```python
from build123d import *

# Parameters (mm, degrees)
MAIN_DEPTH            = 5
GEAR_AXIS_HOLES_D     = 5.5
FILLET1_R             = 3
F_3_CLEARANCE_HOLE1_D = 2.794


with BuildPart() as part:
    # Base → Main (new body)
    with BuildSketch(Plane.XY):
        Polygon((0, 27.5), (-33, 27.5), (-33, -27.5), (0, -27.5), (0, -40.995), (24, -40.995), (31.5, -40.995), (31.5, 27.5), (24, 27.5), align=None)
    extrude(amount=MAIN_DEPTH)

    # Gear Axis Holes (through all)
    with Locations(Plane(origin=(0, 0, 0), x_dir=(-1, 0, 0), z_dir=(0, 0, -1))):
        with Locations((23, -20), (23, 20)):
            Hole(GEAR_AXIS_HOLES_D / 2)

    # Fillet1
    fillet1_edges = [part.edges().sort_by_distance(p)[0] for p in [
        (31.5, 27.5, 2.5),
        (31.5, -40.995, 2.5),
        (0, -40.995, 2.5),
        (0, -27.5, 2.5),
        (-33, -27.5, 2.5),
        (-33, 27.5, 2.5),
    ]]
    fillet(fillet1_edges, radius=FILLET1_R)

    # #3 Clearance Hole1 (through all)
    with Locations(Plane.XY.offset(5)):
        with Locations((10, 23.75), (27.75, 23.75), (27.75, -37.245), (10, -37.245)):
            Hole(F_3_CLEARANCE_HOLE1_D / 2)


solid = part.part
```
Can you work these out from the model? Positions are in its coordinate system, mm. A direction names the side the tool comes from. Round coordinates to 2 decimals unless told otherwise and drop trailing zeros. Loops run counter-clockwise (first coordinate to the right, second up) from the corner with the lowest first, then second, coordinate; pieces in that order, holes last. Notation, with made-up numbers: (73, 37.25) -> (95, 37.25) arc R15 ccw to (95, 54.25) -> close; hole circle Ø6 at (8, 42.25). An arc over 180 degrees is marked (long way). One line per item, written item: value. Start each with the question number.
1. If we mould it in two halves opening along X, with no side actions, what happens to faces 3 (the cylindrical face through (30.645, -40.093, 2.535)), 4 (the cylindrical face through (26.46, -37.78, 2.47)), 5 (the flat face through (-33, 0, 2))? For each: pulls with the +X half, pulls with the -X half, needs draft (parallel to the pull), parting line crosses it, or undercut.
2. For pin 1 (1.5 mm diameter, centred on y = -35.5, z = 1.5, fed in from -X), with a flat end and sliding along its axis, tell me the tip position at first contact or that it passes through.
3. If I drill on probe 1 along Y at (x, z) = (-23, 2.95); probe 2 along Y at (x, z) = (10, 3.5) (3 decimals); probe 3 along X at (y, z) = (21.5, 3.65), over which ranges is the centre line in solid material (lowest first)?
4. If we section it at C-C, the plane z = 2.1: Write out the boundary of the cut face in (x, y) (3 decimals), then the cut area to 3 significant figures.
5. If we section it at A-A, the plane y = -20: Write out the boundary of the cut face in (x, z).
6. For faces 1 (the flat face through (-1, 1, 0)), 2 (the flat face through (0, -34, 2)), which set-ups out of +Z, -Z, +X, -X, +Y, -Y let a thin tool reach every point of the face, with its end or its side?
7. If we section it at B-B, the plane x = -23: Write out the boundary of the cut face in (y, z), then the cut area to 3 significant figures.
Calculated:
1. face 3: pulls with the +X half
1. face 4: undercut
1. face 5: pulls with the -X half
2. pin 1: stops at x = 0
3. probe 1: y = -27.5 to -22.75, -17.25 to 17.25, 22.75 to 27.5
3. probe 2: y = -40.995 to -38.642, -35.848 to 22.353, 25.147 to 27.5
3. probe 3: x = -33 to -25.3, -20.7 to 31.5
4. outline: (-33, -24.5) arc R3 ccw to (-30, -27.5) -> (-3, -27.5) arc R3 cw to (0, -30.5) -> (0, -37.995) arc R3 ccw to (3, -40.995) -> (28.5, -40.995) arc R3 ccw to (31.5, -37.995) -> (31.5, 24.5) arc R3 ccw to (28.5, 27.5) -> (-30, 27.5) arc R3 ccw to (-33, 24.5) -> close; hole circle Ø5.5 at (-23, -20); hole circle Ø5.5 at (-23, 20); hole circle Ø2.794 at (10, -37.245); hole circle Ø2.794 at (10, 23.75); hole circle Ø2.794 at (27.75, -37.245); hole circle Ø2.794 at (27.75, 23.75)
4. area: 3,890 mm²
5. outline: (-33, 0) -> (-25.75, 0) -> (-25.75, 5) -> (-33, 5) -> close; (-20.25, 0) -> (31.5, 0) -> (31.5, 5) -> (-20.25, 5) -> close
6. face 1: -Z, +X, -X, +Y, -Y
6. face 2: +Z, -Z, -X, -Y
7. outline: (-27.5, 0) -> (-22.75, 0) -> (-22.75, 5) -> (-27.5, 5) -> close; (-17.25, 0) -> (17.25, 0) -> (17.25, 5) -> (-17.25, 5) -> close; (22.75, 0) -> (27.5, 0) -> (27.5, 5) -> (22.75, 5) -> close
7. area: 220 mm²
